Input: part model. Units: mm. Frame: model coordinates. Face numbers are marked on the shaded views. A direction names the side the tool comes from. Give positions to 0.01 mm unless a question says otherwise; leave off trailing zeros. Write each loop counter-clockwise with the first axis right and the second up, starting at its lowest first coordinate (ties: lowest second). Pieces come first, ordered by that corner, then holes. Notation, with made-up numbers: (-17.5, 81.25) - (38.5, 81.25) arc R30 ccw to (38.5, 109.25) - close; hole circle Ø9 at (73.5, 7). An arc over 180 degrees is marked (long way). Use a Markdown table: item, result. Add a question column.
1. Set-up query: the marked faces 4, 5, 6 and 7. Return all of +Z, -Z, +X, -X, +Y, -Y with unobstructed straight access to the full face (end or side cutting, diameter ignored); none if empty.
2. Pin query (flat end, axial travel): pin 1 (5 mm diameter, centred on x = 41.5, z = 11, fed in from +Y); pin 2 (3 mm diameter, centred on x = -35, z = 4, fed in from -Y); pin 3 (1 mm diameter, centred on x = -4.5, z = 21, fed in from +Y). Return the tip coordinate at first contact, or that it passes through.
3. Material intervals for probe 1 along Y at (x, z) = (0, 12.5); probe 2 along X at (y, z) = (-13.5, 18.25); probe 3 along X at (y, z) = (59.5, 13.25), sorted ascending.
4. Section query C-C, the plane x = 17.5. Return loops of the section in (y, z), plus the area to 3 significant figures.
5. Mould query, pull axis Y, two halves, no side actions, for the marked faces 1, 2 and 3. Classes: released by +Y, released by -Y, zero draft, split by the parting line, or undercut.
6. Section query D-D, the plane x = 46. Return loops of the section in (y, z), plus the area to 3 significant figures.
7. Section query A-A, the plane y = 0. Return loops of the section in (x, z).
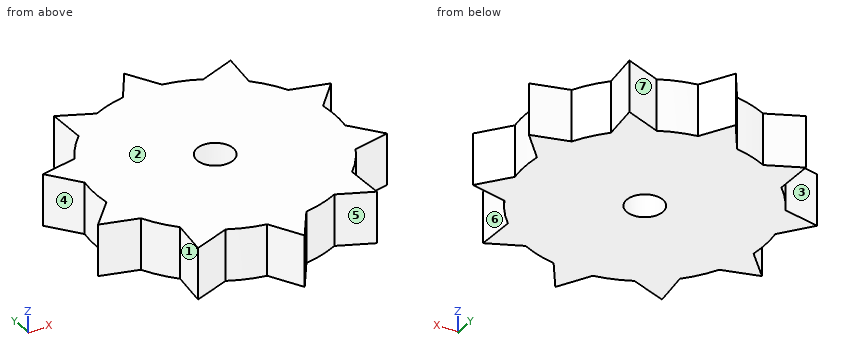
```python
from build123d import *

# Parameters (mm, degrees)
F0_R     = 8.924881
F1_DEPTH = 25.4


with BuildPart() as f1:
    # F0 (on Top) → F1 (new body)
    with BuildSketch(Plane.XY):
        with BuildLine():
            Line((0, 73.399357), (-10.024788, 57.810382))
            ThreePointArc((-10.024788, 57.810382), (-18.123263, 55.803978), (-25.855271, 52.669172))
            Line((-25.855271, 52.669172), (-42.100142, 60.125234))
            Line((-42.100142, 60.125234), (-41.370499, 41.605511))
            ThreePointArc((-41.370499, 41.605511), (-47.193789, 34.860908), (-51.928579, 27.312257))
            Line((-51.928579, 27.312257), (-69.446667, 23.761863))
            Line((-69.446667, 23.761863), (-57.942551, 9.230248))
            ThreePointArc((-57.942551, 9.230248), (-58.672093, 0.349475), (-58.048394, -8.53936))
            Line((-58.048394, -8.53936), (-70.108395, -21.731974))
            Line((-70.108395, -21.731974), (-52.250248, -26.691726))
            ThreePointArc((-52.250248, -26.691726), (-47.605717, -34.296244), (-41.863184, -41.109737))
            Line((-41.863184, -41.109737), (-43.831057, -58.875327))
            Line((-43.831057, -58.875327), (-26.480851, -52.357437))
            ThreePointArc((-26.480851, -52.357437), (-18.246902, -55.763673), (-9.592097, -57.883748))
            Line((-9.592097, -57.883748), (-0.711689, -73.395907))
            Line((-0.711689, -73.395907), (9.46378, -57.904866))
            ThreePointArc((9.46378, -57.904866), (18.123263, -55.803978), (26.364742, -52.416))
            Line((26.364742, -52.416), (42.681144, -59.714199))
            Line((42.681144, -59.714199), (41.771966, -41.202421))
            ThreePointArc((41.771966, -41.202421), (47.529586, -34.401673), (52.190961, -26.807467))
            Line((52.190961, -26.807467), (69.6738, -23.087383))
            Line((69.6738, -23.087383), (58.029324, -8.667996))
            ThreePointArc((58.029324, -8.667996), (58.672724, 0.219434), (57.962866, 9.101802))
            Line((57.962866, 9.101802), (69.894383, 22.410732))
            Line((69.894383, 22.410732), (51.988986, 27.197096))
            ThreePointArc((51.988986, 27.197096), (47.270938, 34.756223), (41.462611, 41.513715))
            Line((41.462611, 41.513715), (43.258134, 59.297551))
            Line((43.258134, 59.297551), (25.971943, 52.611737))
            ThreePointArc((25.971943, 52.611737), (17.705353, 55.937976), (9.030398, 57.974034))
            Line((9.030398, 57.974034), (0, 73.399357))
        make_face()
        Circle(F0_R, mode=Mode.SUBTRACT)
    extrude(amount=F1_DEPTH)


solid = f1.part
```
Result sheet:
| question | item | result |
|---|---|---|
| 1 | face 4 | +Z, -Z, -X |
| 1 | face 5 | +Z, -Z, -Y |
| 1 | face 6 | +Z, -Z, +X |
| 1 | face 7 | +Z, -Z, +Y |
| 2 | pin 1 | stops at y = 59.3 |
| 2 | pin 2 | stops at y = -56.12 |
| 2 | pin 3 | stops at y = 67.18 |
| 3 | probe 1 | y = -72.31 to -8.92, 8.92 to 73.4 |
| 3 | probe 2 | x = -62.58 to 61.93 |
| 3 | probe 3 | x = -42.08 to -40.74, -8.94 to 8.14 |
| 4 | outline | (-56, 0) - (56, 0) - (56, 25.4) - (-56, 25.4) - close |
| 4 | area | 2,840 mm² |
| 5 | face 1 | undercut |
| 5 | face 2 | zero draft |
| 5 | face 3 | released by +Y |
| 6 | outline | (-36.42, 0) - (36.42, 0) - (36.42, 25.4) - (-36.42, 25.4) - close |
| 6 | area | 1,850 mm² |
| 7 | outline | (-58.67, 0) - (-8.92, 0) - (-8.92, 25.4) - (-58.67, 25.4) - close; (8.92, 0) - (58.67, 0) - (58.67, 25.4) - (8.92, 25.4) - close |
